CAD build for the part. Positions are in the model's coordinates, mm. A direction names the side the tool comes from. Round coordinates to 2 decimals unless told otherwise and drop trailing zeros. Loops run counter-clockwise (first coordinate to the right, second up) from the corner with the lowest first, then second, coordinate; pieces in that order, holes last. Notation, with made-up numbers: M -31.5,-37.5 L 25.5,-37.5 A19 ccw 25.5,-3.5 Z; hole C -3.75,73.5 d5. An arc over 180 degrees is marked long. Use a Markdown table: item, result. Add a question column.
(1) Which spindle directions (+Z, -Z, +X, -X, +Y, -Y) get a long thin tool onto all of the face, cutting with end or side? Do faces 1 (the face through (0, -5, -2)), 2 (the face through (-6.583, 0.986, -5.332)). Say none if no direction does.
(2) Band-saw the part on A-A, the plane y = -1.25. Write the cut outline in (x, z).
(3) Wall check: L1, parallel to Z at x = 0, y = -0.75; L2, parallel to Y at x = -7, z = 18; L3, parallel to X at y = -1, z = -1. Give the ranges that are in metal, low to high.
(4) Flat gauge pins, fed straight in: P1, Ø1, axis at x = 9.5, y = 1, coming from the +Z side; P2, Ø3, axis at x = 13, z = -8, coming from the -Y side; P3, Ø8, axis at x = -7.5, z = 11.5, coming from the -Y side; P4, Ø0.6, axis at x = 8.5, y = 1, coming from the -Z side. Where does each tip first touch, or does it go through?
(5) Two-plate mould, pull along Z, no slides. Class faces 3 (the face through (8.131, 0.986, -15.496)), 4 (the face through (3.233, -2.465, -1.341)), 5 (the face through (4, 0, 0)), 6 (the face through (8, 1, -3.947)): released by +Z, released by -Z, zero draft, split by the parting line, or undercut.
(6) Band-saw the part on B-B, the plane z = -9.5. Give the number of separate pieces and of enclosed holes in the cut face, and give its area (3 significant figures).
from build123d import *

# Parameters (mm, degrees)
F2_R     = 1.5
F2_R_2   = 17.5
F2_R_3   = 3.5
F3_DEPTH = 500
F5_DEPTH = 2
F6_DEPTH = 5025
F7_DEPTH = 5


with BuildPart() as f1:
    # F0 (on Top) → F1 (revolve)
    with BuildSketch(Plane.XY):
        with BuildLine():
            Line((-20, 0), (0, 0))
            Line((0, 0), (0, 2))
            Line((0, 2), (-20, 2))
            add(Edge.make_bspline(
                [(-20, 2), (-20.24486, 1.67319), (-20.903414, 0.985438), (-20.240018, 0.339687), (-20, 0)],
                knots=[0, 0, 0, 0, 1.159564, 2.304977, 2.304977, 2.304977, 2.304977], degree=3))
        make_face()
    revolve(axis=Axis((0, 1, 0), (0, -1, 0)))

    # F2 (on Front) → F3 (cut, symmetric)
    with BuildSketch(Plane.XZ):
        Circle(F2_R)
        Circle(F2_R_2)
        Circle(F2_R_3, mode=Mode.SUBTRACT)
    extrude(amount=F3_DEPTH, both=True, mode=Mode.SUBTRACT)

    # F4 (on Front) → F5 (join)
    with BuildSketch(Plane.XZ):
        Polygon((-2.813901, 3.125692), (-10.89626, -15.010192), (-6.329258, -17.045502), (-0.491874, -3.947084), (18.91508, -3.947084), (18.91508, 1.052916), (3.999229, 1.052916), (-5.120873, 17.862287), (-9.515686, 15.477835), align=None)
    extrude(amount=-F5_DEPTH)

    # F2 (on Front) → F6 (cut, symmetric)
    with BuildSketch(Plane.XZ):
        Circle(F2_R)
    extrude(amount=F6_DEPTH, both=True, mode=Mode.SUBTRACT)

    # F2 (on Front) → F7 (join)
    with BuildSketch(Plane.XZ):
        Circle(F2_R_3)
        Circle(F2_R, mode=Mode.SUBTRACT)
    extrude(amount=F7_DEPTH)


solid = f1.part
Return value:
| question | item | result |
|---|---|---|
| 1 | face 1 | +Z, -Z, +X, -X, -Y |
| 1 | face 2 | +Y, -Y |
| 2 | outline | C 0,0 d7; hole C 0,0 d3 |
| 3 | L1 | -3.5 to -1.5, 1.5 to 3.5 |
| 3 | L2 | 0 to 2 |
| 3 | L3 | -3.35 to -1.12, 1.12 to 3.35 |
| 4 | P1 | z = 18.5 |
| 4 | P2 | through |
| 4 | P3 | y = 0 |
| 4 | P4 | z = -18.87 |
| 5 | face 3 | undercut |
| 5 | face 4 | split by the parting line |
| 5 | face 5 | zero draft |
| 5 | face 6 | undercut |
| 6 | separate pieces | 3 |
| 6 | enclosed holes | 0 |
| 6 | area | 24.1 mm^2 |
